from build123d import *

# Parameters (mm, degrees)
F0_R     = 25
F1_DEPTH = 5
F2_R     = 5
F3_DEPTH = 40
F5_R     = 1.5
F6_DEPTH = 40


with BuildPart() as f1:
    # F0 (on Top) → F1 (new body)
    with BuildSketch(Plane.XY):
        Circle(F0_R)
    extrude(amount=F1_DEPTH)

    # F2 (on face) → F3 (join)
    with BuildSketch(Plane.XY.offset(5)):
        Circle(F2_R)
    extrude(amount=F3_DEPTH)

    # F5 (on face) → F6 (join)
    with BuildSketch(Plane.XY.offset(5)):
        with Locations((0, 15)):
            Circle(F5_R)
        with Locations((12.990381, -7.5)):
            Circle(F5_R)
        with Locations((-12.990381, -7.5)):
            Circle(F5_R)
    extrude(amount=F6_DEPTH)


solid = f1.part
Build history of the part. All positions in model axes, mm. A direction names the side the tool comes from. Coordinates: 2 decimals unless noted, no trailing zeros. Order: outer loops, then holes, each group sorted by start corner. A loop starts at its lowest first (then second) coordinate and runs counter-clockwise, first axis right, second up. Notation, with made-up numbers: (25.5, 58) - (41.5, 58) arc R25 cw to (41.5, 94) - close; hole circle Ø7 at (15, 63). An arc over 180 degrees is marked (long way). Write each question's results on one line, items separated by ' | '. Start each with the question number.
Item 1: Mould opens along X. For faces 3 (the face through (0, 0, 0)), 4 (the face through (23.846, 7.509, 2.465)), 5 (the face through (-12.3, -8.83, 24.72)) say: released by +X, released by -X, zero draft, split by the parting line, or undercut.
Item 2: Band-saw the part on B-B on z = 36. Write the cut outline in (x, y).
Item 3: Band-saw the part on A-A on y = 0. Write the cut outline in (x, z).
Item 4: Band-saw the part on C-C on x = 0. Write the cut outline in (y, z).
Item 5: Flat gauge pins, fed straight in: pin 1 (5 mm diameter, centred on y = 1.5, z = 36.5, fed in from +X); pin 2 (8 mm diameter, centred on x = -7.5, y = 7.5, fed in from +Z). Where does each tip first touch, or does it go through?
Item 6: Wall check: probe 1 along Z at (x, y) = (2, 12); probe 2 along X at (y, z) = (-8, 23.5); probe 3 along X at (y, z) = (21.5, 3). Give the ranges that are in metal, low to high. Write a range as [from, to].
Item 7: Band-saw the part on D-D on y = 15. Write the cut outline in (x, z), and give its area (3 significant figures).
Item 8: Tool access for faces 1 (the face through (13, -7, 45)), 2 (the face through (14.38, -8.07, 24.72)): list every direction of +Z, -Z, +X, -X, +Y, -Y with a clear straight run to the whole face (end or side of a thin tool).
Numbers:
1) face 3: zero draft | face 4: split by the parting line | face 5: undercut
2) outline: circle Ø3 at (-12.99, -7.5); circle Ø10 at (0, 0); circle Ø3 at (0, 15); circle Ø3 at (12.99, -7.5)
3) outline: (-25, 0) - (25, 0) - (25, 5) - (5, 5) - (5, 45) - (-5, 45) - (-5, 5) - (-25, 5) - close
4) outline: (-25, 0) - (25, 0) - (25, 5) - (16.5, 5) - (16.5, 45) - (13.5, 45) - (13.5, 5) - (5, 5) - (5, 45) - (-5, 45) - (-5, 5) - (-25, 5) - close
5) pin 1: x = 5 | pin 2: z = 5
6) probe 1: [0, 5] | probe 2: [-14.4, -11.58], [11.58, 14.4] | probe 3: [-12.76, 12.76]
7) outline: (-20, 0) - (20, 0) - (20, 5) - (1.5, 5) - (1.5, 45) - (-1.5, 45) - (-1.5, 5) - (-20, 5) - close | area: 320 mm^2
8) face 1: +Z, +X, -X, +Y, -Y | face 2: +Z
